```python
from build123d import *

# Parameters (mm, degrees)
SKETCH1_R                                      = 340
SKETCH1_R_2                                    = 250
BOSS_EXTRUDE1_DEPTH                            = 12
SKETCH7_W                                      = 30
SKETCH7_H                                      = 12
CUT_EXTRUDE2_DEPTH                             = 12
CIRPATTERN3_COUNT                              = 3
BOSS_EXTRUDE3_DEPTH                            = 12
SKETCH9_W                                      = 60
SKETCH9_H                                      = 70
CUT_EXTRUDE3_DEPTH                             = 12
CUT_EXTRUDE4_DEPTH                             = 12
CIRPATTERN4_COUNT                              = 3
SKETCH11_R                                     = 2
CUT_EXTRUDE5_DEPTH                             = 12
FILLET1_R                                      = 30
CSK_FOR_M4_FLAT_HEAD_MACHINE_SCREW_D           = 4.5
CSK_FOR_M4_FLAT_HEAD_MACHINE_SCREW_CSINK_D     = 9.4
CSK_FOR_M4_FLAT_HEAD_MACHINE_SCREW_CSINK_ANGLE = 90


with BuildPart() as part:
    # Sketch1 → Boss-Extrude1 (new body)
    with BuildSketch(Plane(origin=(0, 82.464823413, 0), x_dir=(1, 0, 0), z_dir=(0, 1, 0))):
        Circle(SKETCH1_R)
        Circle(SKETCH1_R_2, mode=Mode.SUBTRACT)
    extrude(amount=-BOSS_EXTRUDE1_DEPTH)

    # Sketch7 → Cut-Extrude2 (cut)
    with BuildSketch(Plane.XZ.offset(-70.464823413)):
        with Locations((60, 272.5)):
            Rectangle(SKETCH7_W, SKETCH7_H)
        with Locations((-60, 272.5)):
            Rectangle(SKETCH7_W, SKETCH7_H)
    cut_extrude2 = extrude(amount=-CUT_EXTRUDE2_DEPTH, mode=Mode.SUBTRACT)

    # CirPattern3: Cut-Extrude2 ×3 about axis
    cirpattern3_axis = Axis((0, 0, 0), (0, 1, 0))
    for i in range(1, CIRPATTERN3_COUNT):
        add(cut_extrude2.rotate(cirpattern3_axis, i * 360 / CIRPATTERN3_COUNT), mode=Mode.SUBTRACT)

    # Sketch8 → Boss-Extrude3 (add)
    with BuildSketch(Plane(origin=(0, 82.464823413, 0), x_dir=(1, 0, 0), z_dir=(0, 1, 0))):
        with BuildLine():
            Line((-40, -420), (40, -420))
            Line((40, -420), (226.378812173, -253.678208364))
            ThreePointArc((226.378812173, -253.678208364), (0, -340), (-226.378812173, -253.678208364))
            Line((-226.378812173, -253.678208364), (-40, -420))
        make_face()
    extrude(amount=-BOSS_EXTRUDE3_DEPTH)

    # Sketch9 → Cut-Extrude3 (cut)
    with BuildSketch(Plane(origin=(0, 82.464823413, 0), x_dir=(1, 0, 0), z_dir=(0, 1, 0))):
        with Locations((0, -345)):
            Rectangle(SKETCH9_W, SKETCH9_H)
    extrude(amount=-CUT_EXTRUDE3_DEPTH, mode=Mode.SUBTRACT)

    # Sketch10 → Cut-Extrude4 (cut)
    with BuildSketch(Plane(origin=(0, 82.464823413, 0), x_dir=(1, 0, 0), z_dir=(0, 1, 0))):
        Polygon((233.219163867, -160.052558883), (255.219163867, -121.947441117), (291.592230826, -142.947441117), (269.592230826, -181.052558883), align=None)
    cut_extrude4 = extrude(amount=-CUT_EXTRUDE4_DEPTH, mode=Mode.SUBTRACT)

    # CirPattern4: Cut-Extrude4 ×3 about axis
    cirpattern4_axis = Axis((0, 0, 0), (0, 1, 0))
    for i in range(1, CIRPATTERN4_COUNT):
        add(cut_extrude4.rotate(cirpattern4_axis, i * 360 / CIRPATTERN4_COUNT), mode=Mode.SUBTRACT)

    # Sketch11 → Cut-Extrude5 (cut)
    with BuildSketch(Plane(origin=(0, 82.464823413, 0), x_dir=(1, 0, 0), z_dir=(0, 1, 0))):
        with Locations((-45, -365)):
            Circle(SKETCH11_R)
        with Locations((-45, -325)):
            Circle(SKETCH11_R)
        with Locations((45, -365)):
            Circle(SKETCH11_R)
        with Locations((45, -325)):
            Circle(SKETCH11_R)
    extrude(amount=-CUT_EXTRUDE5_DEPTH, mode=Mode.SUBTRACT)

    # Fillet1
    fillet1_edges = [part.edges().sort_by_distance(p)[0] for p in [
        (-40, 76.464823413, 420),
        (40, 76.464823413, 420),
    ]]
    fillet(fillet1_edges, radius=FILLET1_R)

    # CSK for M4 Flat Head Machine Screw (through all)
    with Locations(Plane(origin=(0, 82.464823413, 0), x_dir=(1, 0, 0), z_dir=(0, 1, 0))):
        with Locations((80.233903982, 299.43700615), (219.203102168, 219.203102168), (299.43700615, 80.233903982), (299.43700615, -80.233903982), (219.203102168, -219.203102168), (80.233903982, -299.43700615), (-80.233903982, -299.43700615), (-219.203102168, -219.203102168), (-299.43700615, -80.233903982), (-299.43700615, 80.233903982), (-219.203102168, 219.203102168), (-80.233903982, 299.43700615), (0, 0)):
            CounterSinkHole(CSK_FOR_M4_FLAT_HEAD_MACHINE_SCREW_D / 2, CSK_FOR_M4_FLAT_HEAD_MACHINE_SCREW_CSINK_D / 2, counter_sink_angle=CSK_FOR_M4_FLAT_HEAD_MACHINE_SCREW_CSINK_ANGLE)


solid = part.part
```
The listing builds one solid part. Answer for the finished solid, in the listing's coordinates (mm). A direction names the side the tool comes from. Round coordinates to 2 decimals unless told otherwise and drop trailing zeros. Loops run counter-clockwise (first coordinate to the right, second up) from the corner with the lowest first, then second, coordinate; pieces in that order, holes last.
1) For faces 4 (the face through (-138.7, 76.55, 331.92)), 5 (the face through (251.66, 76.55, 170.7)), determine the directions among +Z, -Z, +X, -X, +Y, -Y from which every point of the face is accessible in a straight line to the end or side of a thin tool.
Outcome:
face 4: +Z, -X, +Y, -Y
face 5: +Y, -Y
2) A cutting plane is placed at C-C on x = -143. Determine the outline of the cut face in (y, z).
Outcome:
outline: (70.46, -308.47) - (82.46, -308.47) - (82.46, -205.06) - (70.46, -205.06) - close; (70.46, 205.06) - (82.46, 205.06) - (82.46, 328.08) - (70.46, 328.08) - close
3) A cutting plane is placed at A-A on z = 0. Determine the outline of the cut face in (x, y).
Outcome:
outline: (-340, 70.46) - (-250, 70.46) - (-250, 82.46) - (-340, 82.46) - close; (250, 70.46) - (340, 70.46) - (340, 82.46) - (250, 82.46) - close
4) A cutting plane is placed at D-D on y = 73. Give the number of separate pieces and of enclosed holes in the cut face, plus the area to 3 significant figures.
Outcome:
separate pieces: 1
enclosed holes: 27
area: 172,000 mm2
5) A cutting plane is placed at B-B on x = 0. Determine the outline of the cut face in (y, z), plus the area to 3 significant figures.
Outcome:
outline: (70.46, -340) - (82.46, -340) - (82.46, -324) - (70.46, -324) - close; (70.46, -282) - (82.46, -282) - (82.46, -250) - (70.46, -250) - close; (70.46, 250) - (82.46, 250) - (82.46, 310) - (70.46, 310) - close; (70.46, 380) - (82.46, 380) - (82.46, 420) - (70.46, 420) - close
area: 1,780 mm2
6) Given P1, Ø3.5, axis at x = -7, y = 75, coming from the -Z side; P2, Ø2.5, axis at x = 299.44, z = 80.23, coming from the +Y side; P3, Ø5, axis at y = 73, z = 223, coming from the -X side; P4, Ø5, axis at x = 219.2, z = 219.2, coming from the -Y side, each flat-ended and moving along its own axis, determine where each tip first touches the part or whether it passes through.
Outcome:
P1: stops at z = -339.96
P2: passes through
P3: stops at x = -258.8
P4: stops at y = 70.46
7) Consider line 1 (Z direction, x = -8.5, y = 77.5); line 2 (Z direction, x = -47.5, y = 79.5); line 3 (Z direction, x = -62.5, y = 76). Determine where each line is inside the solid, lowest interval first.
Outcome:
line 1: z = -339.89 to -324, -282 to -249.86, 249.86 to 310, 380 to 420
line 2: z = -336.67 to -245.45, 245.45 to 266.5, 278.5 to 413.27
line 3: z = -334.21 to -242.06, 242.06 to 266.5, 278.5 to 399.92
8) For a pull along Z with two mould halves and no side action, classify faces 1 (the face through (136.212, 76.549, 334.142)), 2 (the face through (-244.373, 76.549, 140.733)), 3 (the face through (146, 70.465, 204)) as released by +Z, released by -Z, zero draft, split by the parting line, or undercut.
Outcome:
face 1: released by +Z
face 2: undercut
face 3: zero draft
